```python
from build123d import *

# Parameters (mm, degrees)
F1_DEPTH      = 4
F1_DEPTH_BACK = 4
F3_DEPTH      = 10
F5_DEPTH      = 25
F7_DEPTH      = 21.7


with BuildPart() as f1:
    # F0 (on Front) → F1 (new body, two sides)
    with BuildSketch(Plane.XZ) as f1_sk:
        Polygon((-10.85, 10.85), (-10.85, 0), (-10.85, -10.85), (0, -10.85), (10.85, -10.85), (10.85, 0), (10.85, 10.85), (0, 10.85), align=None)
        Polygon((8.85, 8.85), (8.85, 0), (8.85, -8.85), (0, -8.85), (-8.85, -8.85), (-8.85, 0), (-8.85, 8.85), (0, 8.85), align=None, mode=Mode.SUBTRACT)
    extrude(amount=F1_DEPTH)
    extrude(f1_sk.sketch, amount=-F1_DEPTH_BACK)

    # F2 (on face) → F3 (join)
    with BuildSketch(Plane.XY.offset(10.85)):
        Polygon((-14.7346977867, 1.2544146994), (-10.85, -1.1231439692), (-10.85, 4), (8.7051686149, 4), (1.0543529996, 13.7034736867), align=None)
        Polygon((-6.1494992707, -4), (10.1865680069, -4), (10.85, -3.4769094021), (10.85, 1.2797259855), (8.7051686149, 4), (-10.85, 4), (-10.85, -1.1231439692), align=None)
        Polygon((-6.1494992707, -4), (3.047517268, -9.6288667992), (10.1865680069, -4), align=None)
        Polygon((10.85, 1.2797259855), (10.85, -3.4769094021), (13.1626902148, -1.6534421593), align=None)
    extrude(amount=F3_DEPTH)

    # F4 (on Right) → F5 (cut)
    with BuildSketch(Plane.YZ):
        Polygon((-36.6991721094, 6.3178054057), (17.9703272879, 21.0884753615), (-36.6991721094, 33.6725451052), align=None)
    extrude(amount=-F5_DEPTH, mode=Mode.SUBTRACT)

    # F6 (on face) → F7 (cut)
    with BuildSketch(Plane(origin=(0, 0, -10.85), x_dir=(1, 0, 0), z_dir=(0, 0, -1))):
        with BuildLine():
            Line((13.9217844345, 4.8126999282), (9.694906495, 4.8126999282))
            ThreePointArc((9.694906495, 4.8126999282), (9.8845588749, 4.4100780486), (10.0574993187, 4))
            Line((10.0574993187, 4), (10.85, 4))
            Line((10.85, 4), (10.85, -4))
            Line((10.85, -4), (10.0574993187, -4))
            ThreePointArc((10.0574993187, -4), (9.8311449192, -4.52790041), (9.5771050518, -5.0430498086))
            Line((9.5771050518, -5.0430498086), (13.9217844345, -5.0430498086))
            Line((13.9217844345, -5.0430498086), (13.9217844345, 4.8126999282))
        make_face()
        with BuildLine():
            Line((10.85, 4), (10.0574993187, 4))
            ThreePointArc((10.0574993187, 4), (10.6304521223, 2.0363644618), (10.8237374574, 0))
            ThreePointArc((10.8237374574, 0), (10.6304521223, -2.0363644618), (10.0574993187, -4))
            Line((10.0574993187, -4), (10.85, -4))
            Line((10.85, -4), (10.85, 4))
        make_face()
        with BuildLine():
            ThreePointArc((-10.0574993187, -4), (-10.8237374574, 0), (-10.0574993187, 4))
            Line((-10.0574993187, 4), (-10.85, 4))
            Line((-10.85, 4), (-10.85, -4))
            Line((-10.85, -4), (-10.0574993187, -4))
        make_face()
    extrude(amount=-F7_DEPTH, mode=Mode.SUBTRACT)


solid = f1.part
```
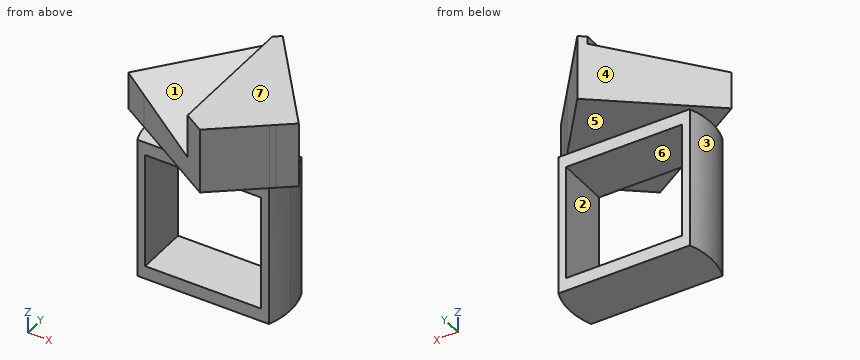
Verification items for the finished model (mm, model axes). Face numbers are marked on the shaded views. A direction names the side the tool comes from. Round coordinates to 2 decimals unless told otherwise and drop trailing zeros. Loops run counter-clockwise (first coordinate to the right, second up) from the corner with the lowest first, then second, coordinate; pieces in that order, holes last. Notation, with made-up numbers: (-24, 64.25) -> (17, 64.25) arc R21 ccw to (17, 84.25) -> close; hole circle Ø10 at (68, 49). An arc over 180 degrees is marked (long way). Answer as a JSON object with one key per item and string values.
Q1. Go/stop test with flat-tipped pins: P1, Ø9, axis at y = 1, z = -2, coming from the -X side; P2, Ø2.5, axis at x = -8, y = -2.5, coming from the +Z side; P3, Ø9, axis at y = -1.5, z = -4, coming from the +X side. Record where each tip stops, or that it passes through.
Data:
{"P1": "stops at x = -10.82", "P2": "stops at z = 15.9", "P3": "stops at x = 10.82"}
Q2. Access from +Z, -Z, +X, -X, +Y, -Y to the whole of each face (thin tool, end or side, straight path). Record for the marked faces 1, 2, 3 and 4.
Data:
{"face 1": "+Z, -X, -Y", "face 2": "+Y, -Y", "face 3": "-Z, -X", "face 4": "+Z, -Z, -X, +Y"}
Q3. Section check D-D (z = 12). Record the boundary of the cut face in (x, y), then the cut area to 3 significant figures.
Data:
{"outline": "(-14.73, 1.25) -> (3.05, -9.63) -> (13.16, -1.65) -> (1.05, 13.7) -> close", "area": "323 mm2"}
Q4. Section check B-B (x = 7). Record the boundary of the cut face in (y, z).
Data:
{"outline": "(-6.51, 10.85) -> (-4, 10.85) -> (-4, 8.85) -> (4, 8.85) -> (4, 10.85) -> (6.16, 10.85) -> (6.16, 20.85) -> (-6.51, 20.85) -> close; (-4, -10.85) -> (4, -10.85) -> (4, -8.85) -> (-4, -8.85) -> close"}
Q5. Section check A-A (z = 7). Record the boundary of the cut face in (x, y), then the cut area to 3 significant figures.
Data:
{"outline": "(-10.06, -4) -> (-8.85, -4) -> (-8.85, 4) -> (-10.06, 4) arc R10.82 ccw to start; (8.85, -4) -> (10.06, -4) arc R10.82 ccw to (10.06, 4) -> (8.85, 4) -> close", "area": "27.6 mm2"}
Q6. Draft check along Z on the marked faces 5, 6 and 7. Enter one of: pulls with the +Z half, pulls with the -Z half, needs draft (parallel to the pull), parting line crosses it, or undercut.
Data:
{"face 5": "pulls with the -Z half", "face 6": "undercut", "face 7": "pulls with the +Z half"}
Q7. Scan lines: line 1 (Z direction, x = 1.75, y = -1.5); line 2 (Z direction, x = -3.75, y = 2.5); line 3 (X direction, y = -1.75, z = -2). Record each from-to range of solid material in increasing order. Write a range as from..to.
Data:
{"line 1": "z = -10.85..-8.85, 8.85..20.85", "line 2": "z = -10.85..-8.85, 8.85..16.91", "line 3": "x = -10.68..-8.85, 8.85..10.68"}
Q8. Section check C-C (y = 2). Record the boundary of the cut face in (x, z).
Data:
{"outline": "(-13.79, 10.85) -> (-10.64, 10.85) -> (-10.64, -10.85) -> (10.64, -10.85) -> (10.64, 10.85) -> (10.28, 10.85) -> (10.28, 20.85) -> (0, 20.85) -> (0, 16.77) -> (-13.79, 16.77) -> close; hole (-8.85, -8.85) -> (8.85, -8.85) -> (8.85, 8.85) -> (-8.85, 8.85) -> close"}
